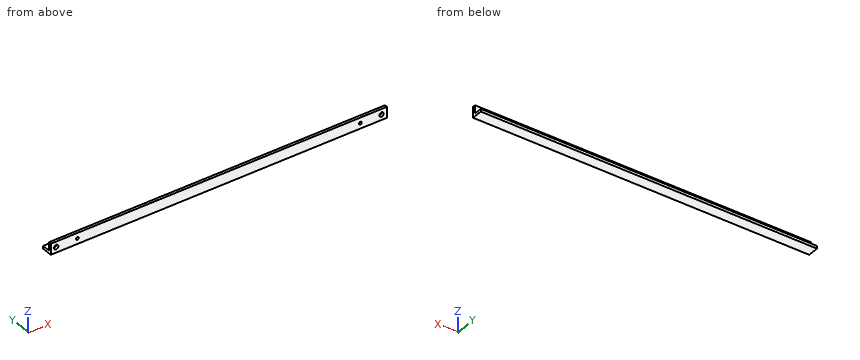
from build123d import *

# Parameters (mm, degrees)
BOSS_EXTRUDE1_DEPTH = 787.4
SKETCH2_R           = 5.08
SKETCH2_R_2         = 3.175
CUT_EXTRUDE1_DEPTH  = 914.4


with BuildPart() as part:
    # Sketch1 → Boss-Extrude1 (new body)
    with BuildSketch(Plane(origin=(0, 0, 0), x_dir=(0, 0, -1), z_dir=(1, 0, 0))):
        Polygon((0, 0), (0, 19.05), (6.35, 19.05), (6.35, -6.35), (-19.05, -6.35), (-19.05, 0), align=None)
    extrude(amount=BOSS_EXTRUDE1_DEPTH)

    # Sketch2 → Cut-Extrude1 (cut)
    with BuildSketch(Plane.XZ.offset(6.35)):
        with Locations(Location((12.7, 6.35, 0), (0, 0, 270))):
            Circle(SKETCH2_R)
        with Locations(Location((62.357, 6.35, 0), (0, 0, 270))):
            Circle(SKETCH2_R_2)
        with Locations(Location((725.043, 6.35, 0), (0, 0, 270))):
            Circle(SKETCH2_R_2)
        with Locations(Location((774.7, 6.35, 0), (0, 0, 270))):
            Circle(SKETCH2_R)
    extrude(amount=-CUT_EXTRUDE1_DEPTH, mode=Mode.SUBTRACT)


solid = part.part
Design review of the part built by this model. Coordinates are the model's own, in mm. Coordinates: 2 decimals unless noted, no trailing zeros. Order: outer loops, then holes, each group sorted by start corner. A loop starts at its lowest first (then second) coordinate and runs counter-clockwise, first axis right, second up.
Item 1: For pin 1 Ø15 at (x, z) = (313.5, 13.5) entering from +Y; pin 2 Ø1 at (y, z) = (-0.5, 15) entering from -X, all flat-tipped, find the tip position at first contact; note any pin that passes through.
Item 2: For line 1 (X direction, y = -3.75, z = 6.35); line 2 (Z direction, x = 774.7, y = -2); line 3 (Y direction, x = 452, z = 7.75), list the stretches that pass through material, from the lowest coordinate up.
Item 3: Take a section at B-B, the plane x = 356. Write out the cut boundary in (y, z).
Item 4: Take a section at A-A, the plane y = 12.5. Write out the cut boundary in (x, z).
The answers:
1. pin 1: stops at y = 0
1. pin 2: stops at x = 0
2. line 1: x = 0 to 7.62, 17.78 to 59.18, 65.53 to 721.87, 728.22 to 769.62, 779.78 to 787.4
2. line 2: z = -6.35 to 1.27, 11.43 to 19.05
2. line 3: y = -6.35 to 0
3. outline: (-6.35, -6.35) - (19.05, -6.35) - (19.05, 0) - (0, 0) - (0, 19.05) - (-6.35, 19.05) - close
4. outline: (0, -6.35) - (787.4, -6.35) - (787.4, 0) - (0, 0) - close
